Geometry check sheet. Reference: drawing and pictorial views, mm from the part's lowest x, y, z. Give positions to 0.01 mm unless a question says otherwise; leave off trailing zeros. Order: outer loops, then holes, each group sorted by start corner. A loop starts at its lowest first (then second) coordinate and runs counter-clockwise, first axis right, second up.
Item 1: Sectioned sample at B-B on y = 25. Record the boundary of the cut face in (x, z).
Item 2: Material ranges on line 1 along Y through (x, z) = (418, 5.75); line 2 along Y through (x, z) = (214, 6); line 3 along X through (y, z) = (20, 8.25), recorded low to high.
Item 3: Gauge pin test, flat end, axial feed: P1, Ø3, axis at x = 92.5, y = 134, coming from the +Z side. Record the tip position at first contact, or that the pin passes through.
Item 4: Sectioned sample at A-A on x = 264. Record the boundary of the cut face in (y, z).
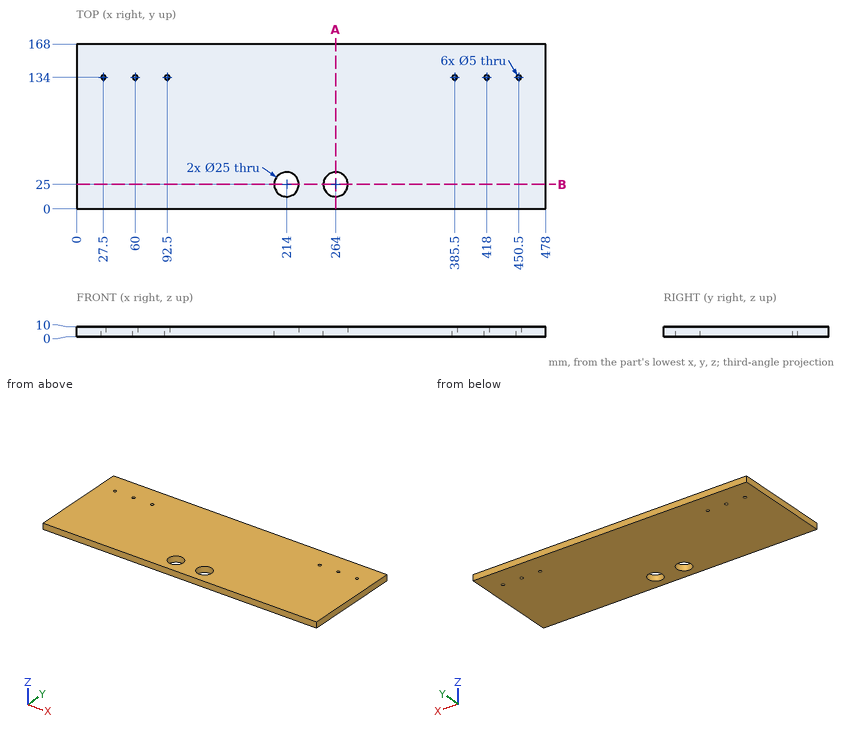
Report:
1. outline: (0, 0) - (201.5, 0) - (201.5, 10) - (0, 10) - close; (226.5, 0) - (251.5, 0) - (251.5, 10) - (226.5, 10) - close; (276.5, 0) - (478, 0) - (478, 10) - (276.5, 10) - close
2. line 1: y = 0 to 131.5, 136.5 to 168
2. line 2: y = 0 to 12.5, 37.5 to 168
2. line 3: x = 0 to 202.54, 225.46 to 252.54, 275.46 to 478
3. P1: passes through
4. outline: (0, 0) - (12.5, 0) - (12.5, 10) - (0, 10) - close; (37.5, 0) - (168, 0) - (168, 10) - (37.5, 10) - close
